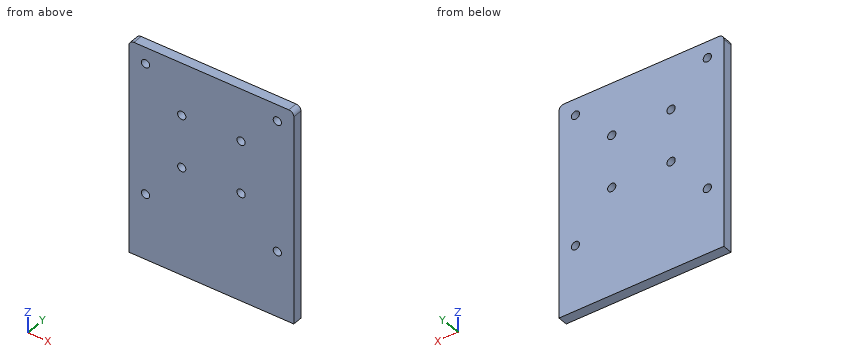
```python
from build123d import *

# Parameters (mm, degrees)
SKETCH1_W           = 100
SKETCH1_H           = 130
SKETCH1_R           = 2.5
BOSS_EXTRUDE1_DEPTH = 6
FILLET1_R           = 3


with BuildPart() as part:
    # Sketch1 → Boss-Extrude1 (new body)
    with BuildSketch(Plane(origin=(0, 0, 0), x_dir=(1, 0, 0), z_dir=(0, 1, 0))):
        with Locations((40, 55)):
            Rectangle(SKETCH1_W, SKETCH1_H)
        Circle(SKETCH1_R, mode=Mode.SUBTRACT)
        with Locations((80, 0)):
            Circle(SKETCH1_R, mode=Mode.SUBTRACT)
        with Locations((0, 80)):
            Circle(SKETCH1_R, mode=Mode.SUBTRACT)
        with Locations((80, 80)):
            Circle(SKETCH1_R, mode=Mode.SUBTRACT)
        with Locations((22, 22)):
            Circle(SKETCH1_R, mode=Mode.SUBTRACT)
        with Locations((58, 22)):
            Circle(SKETCH1_R, mode=Mode.SUBTRACT)
        with Locations((22, 54)):
            Circle(SKETCH1_R, mode=Mode.SUBTRACT)
        with Locations((58, 54)):
            Circle(SKETCH1_R, mode=Mode.SUBTRACT)
    extrude(amount=BOSS_EXTRUDE1_DEPTH)

    # Fillet1
    fillet1_edges = [part.edges().sort_by_distance(p)[0] for p in [
        (90, 3, 10),
        (-10, 3, 10),
    ]]
    fillet(fillet1_edges, radius=FILLET1_R)


solid = part.part
```
The listing builds one solid part. Answer for the finished solid, in the listing's coordinates (mm). Round coordinates to 2 decimals unless told otherwise and drop trailing zeros. Order: outer loops, then holes, each group sorted by start corner. A loop starts at its lowest first (then second) coordinate and runs counter-clockwise, first axis right, second up. Notation, with made-up numbers: (7.5, 67) - (28.5, 67) arc R17 ccw to (28.5, 86) - close; hole circle Ø2 at (14.25, 21.5). An arc over 180 degrees is marked (long way). Put each result on its own line as item: value. Start each with the question number.
(1) Given P1, Ø4.5, axis at x = 22, z = -22, coming from the +Y side, flat-ended and moving along its own axis, determine where the tip first touches the part or whether it passes through.
(2) Straight lines are drawn through the part: probe 1 along Z at (x, y) = (58, 1.8); probe 2 along X at (y, z) = (2.25, -80); probe 3 along Z at (x, y) = (0, 3.8). For each, find the intervals that lie inside material, in ascending order. Write a range as from..to.
(3) Find section A-A (x = 22). Give the vertices of the cut face in (y, z).
(4) Find section B-B (z = -80). Give the vertices of the cut face in (x, y).
Reply:
1. P1: through
2. probe 1: -120..-56.5, -51.5..-24.5, -19.5..10
2. probe 2: -10..-2.5, 2.5..77.5, 82.5..90
2. probe 3: -120..-82.5, -77.5..-2.5, 2.5..10
3. outline: (0, -120) - (6, -120) - (6, -56.5) - (0, -56.5) - close; (0, -51.5) - (6, -51.5) - (6, -24.5) - (0, -24.5) - close; (0, -19.5) - (6, -19.5) - (6, 10) - (0, 10) - close
4. outline: (-10, 0) - (-2.5, 0) - (-2.5, 6) - (-10, 6) - close; (2.5, 0) - (77.5, 0) - (77.5, 6) - (2.5, 6) - close; (82.5, 0) - (90, 0) - (90, 6) - (82.5, 6) - close
